Geometry: final body of the model. Coordinates: model frame, mm. A direction names the side the tool comes from. Give positions to 0.01 mm unless a question says otherwise; leave off trailing zeros. Write each loop counter-clockwise with the first axis right and the second up, starting at its lowest first coordinate (ties: lowest second). Pieces come first, ordered by that corner, then holes.
Autodesk Inventor part; units mm, degrees
ref_plane "Work Plane1" through (8.5, 0, 0) normal (1, 0, 0) x (0, 1, 0)
ref_plane "Work Plane2" through (0, 20, 0) normal (0, 1, 0) x (-1, 0, 0)
ref_plane "XY Plane" through (0, 0, 0) normal (0, 0, 1) x (1, 0, 0)
sketch "Sketch1" plane through (0, 0, 0) normal (0, 0, 1) x (1, 0, 0)
  circle A0 centre (17, 3) radius 1.4
  circle A1 centre (0, 20) radius 1.4
  circle A2 centre (17, 20) radius 1.4
  circle A3 centre (0, 3) radius 1.4
  arc A4 (-1.2644, 15.3609) -> (-1.2644, 7.6391) centre (8.5, 11.5) ccw
  arc A5 (-1.8746, 5.3422) -> (-1.2644, 7.6391) centre (-3.1243, 6.9037) ccw
  arc A6 (-1.8746, 5.3422) -> (0, 0) centre (0, 3) ccw
  line L0 (0, 0) -> (17, 0)
  arc A7 (17, 0) -> (18.8746, 5.3422) centre (17, 3) ccw
  arc A8 (18.2644, 7.6391) -> (18.8746, 5.3422) centre (20.1243, 6.9037) ccw
  arc A9 (18.2644, 7.6391) -> (18.2644, 15.3609) centre (8.5, 11.5) ccw
  arc A10 (18.8746, 17.6578) -> (18.2644, 15.3609) centre (20.1243, 16.0963) ccw
  arc A11 (18.8746, 17.6578) -> (17, 23) centre (17, 20) ccw
  line L1 (17, 23) -> (0, 23)
  arc A12 (0, 23) -> (-1.8746, 17.6578) centre (0, 20) ccw
  arc A13 (-1.2644, 15.3609) -> (-1.8746, 17.6578) centre (-3.1243, 16.0963) ccw
extrude "Extrusion1" add sketch "Sketch1" along normal blind 2.6
sketch "Sketch2" plane through (0, 0, 0) normal (0, 0, -1) x (-1, 0, 0)
  circle A0 centre (-8.5, 11.5) radius 9
extrude "Extrusion2" add sketch "Sketch2" along normal blind 4
sketch "Sketch3" plane through (8.5, 11.5, -4) normal (0, 0, -1) x (-1, 0, 0)
  arc A0 (0, 7.5) -> (-5.3033, 5.3033) centre (0, 0) ccw
  arc A1 (0, 2.5) -> (0, 7.5) centre (0, 5) ccw
  arc A2 (0, 2.5) -> (-1.7678, 1.7678) centre (0, 0) ccw
  arc A3 (-5.3033, 5.3033) -> (-1.7678, 1.7678) centre (-3.5355, 3.5355) ccw
extrude "Extrusion3" cut sketch "Sketch3" against normal blind 4
sketch "Sketch4" plane through (0, 0, 2.6) normal (0, 0, 1) x (1, 0, 0)
  circle A0 centre (8.5, 16.5) radius 3.5
extrude "Extrusion4" add sketch "Sketch4" along normal blind 15
ref_plane "Work Plane1" through (8.5, 0, 0) normal (1, 0, 0) x (0, 1, 0)
sketch "Sketch6" plane through (8.5, 0, 0) normal (1, 0, 0) x (0, 1, 0)
  circle A0 centre (20, 17.6) radius 1
  line L0 (16.5, 17.6) -> (16.5, 21.4909) construction
revolve "Revolution1" add sketch "Sketch6" angle 360 about axis through (8.5, 16.5, 17.6) along (0, 0, 1)
ref_plane "Work Plane2" through (0, 20, 0) normal (0, 1, 0) x (-1, 0, 0)
sketch "Sketch7" plane through (0, 20, 0) normal (0, 1, 0) x (-1, 0, 0)
  circle A0 centre (-8.5, 8.1) radius 3.5
extrude "Extrusion6" add sketch "Sketch7" along normal blind 2 and the other way blind 3.5
sketch "Sketch8" plane through (8.5, 16.5, 17.6) normal (0, 0, 1) x (1, 0, 0)
  circle A0 centre (0, 0) radius 2.5
extrude "Extrusion8" cut sketch "Sketch8" against normal blind 20
sketch "Sketch9" plane through (8.5, 22, 8.1) normal (0, 1, 0) x (1, 0, 0)
  circle A0 centre (0, 0) radius 2
extrude "Extrusion9" cut sketch "Sketch9" against normal blind 5
thread "Thread1"
sketch "Sketch10" plane through (0, 0, 2.6) normal (0, 0, 1) x (1, 0, 0)
  circle A0 centre (8.5, 11.5) radius 1.5
extrude "Extrusion10" cut sketch "Sketch10" against normal blind 10
properties part number "cover"
Item 1: Section C-C, the plane z = 13.5. Return the cut outline in (x, y), plus the area to 3 significant figures.
Found:
outline: circle Ø7 at (8.5, 16.5); hole circle Ø5 at (8.5, 16.5)
area: 18.8 mm2
Item 2: Pull-direction query (X, two-part tool) for faces 1 (the face through (9, 23, 1)), 2 (the face through (19, 11.6, 1.3)), 3 (the face through (12, 15, 0)); classes: +X half, -X half, draft (parallel to the pull), parting line (faces both ways), or undercut.
Found:
face 1: draft
face 2: +X half
face 3: undercut
Item 3: Pin query (flat end, axial travel): pin 1 Ø3 at (x, y) = (0, 3) entering from +Z; pin 2 Ø2.5 at (x, y) = (8.5, 11.5) entering from -Z; pin 3 Ø1.5 at (x, z) = (11, 10.5) entering from -Y. Return the tip coordinate at first contact, or that it passes through.
Found:
pin 1: stops at z = 2.6
pin 2: stops at z = 16.63
pin 3: stops at y = 13.47
Item 4: Section A-A, the plane y = 11. Return the cut outline in (x, z).
Found:
outline: (-1.99, 0) - (-0.49, 0) - (-0.49, -4) - (7.09, -4) - (7.09, 2.6) - (-1.99, 2.6) - close; (9.91, -4) - (17.49, -4) - (17.49, 0) - (18.99, 0) - (18.99, 2.6) - (9.91, 2.6) - close
Item 5: Line query: L1, parallel to Y at x = 8.5, z = -2.25; L2, parallel to Y at x = 17, z = 1.15; L3, parallel to Y at x = 8.5, z = 11.75. Output: solid intervals per line, ascending.
Found:
L1: y = 2.5 to 10, 13 to 14, 19 to 20.5
L2: y = 0 to 1.6, 4.4 to 18.6, 21.4 to 23
L3: y = 13 to 14, 19 to 20
Item 6: Section B-B, the plane z = 8.1. Return the cut outline in (x, y), plus the area to 3 significant figures.
Found:
outline: (5, 16.5) arc R3.5 ccw to (12, 16.5) - (12, 22) - (10.5, 22) - (10.5, 18) arc R2.5 cw (long way) to (6.5, 18) - (6.5, 22) - (5, 22) - close
area: 24.9 mm2
Item 7: Reachability of faces 4 (the face through (9, 22, 6)), 5 (the face through (19.813, 21.042, 1.282)), 6 (the face through (4.347, 19.485, -1.972)), 7 (the face through (8.04, 13.03, 9.5)) from +Z, -Z, +X, -X, +Y, -Y: full face, straight path, thin tool, end or side. Return the list, or none.
Found:
face 4: +Z, +X, -X, +Y
face 5: +Z, -Z, +X
face 6: -Z
face 7: none
Item 8: Section D-D, the plane y = 3. Return the cut outline in (x, z).
Found:
outline: (-3, 0) - (-1.4, 0) - (-1.4, 2.6) - (-3, 2.6) - close; (1.4, 0) - (5.54, 0) - (5.54, -4) - (11.46, -4) - (11.46, 0) - (15.6, 0) - (15.6, 2.6) - (1.4, 2.6) - close; (18.4, 0) - (20, 0) - (20, 2.6) - (18.4, 2.6) - close
